Autodesk Inventor part; units mm, degrees
ref_plane "YZ Plane" through (0, 0, 0) normal (1, 0, 0) x (0, 1, 0)
ref_plane "XZ Plane" through (0, 0, 0) normal (0, 1, 0) x (-1, 0, 0)
ref_plane "XY Plane" through (0, 0, 0) normal (0, 0, 1) x (1, 0, 0)
sketch "Sketch1" plane through (0, 0, 0) normal (0, 0, 1) x (1, 0, 0)
  line L0 (57.5, 0) -> (28.75, -49.7965)
  line L1 (28.75, -49.7965) -> (-28.75, -49.7965)
  line L2 (-28.75, -49.7965) -> (-57.5, 0)
  line L3 (-57.5, 0) -> (-28.75, 49.7965)
  line L4 (-28.75, 49.7965) -> (28.75, 49.7965)
  line L5 (28.75, 49.7965) -> (57.5, 0)
  point P0 (0, 0)
  point P1 (0, 0)
  dimension "d0" = 115
extrude "Extrusion1" add sketch "Sketch1" along normal blind 159.4929
sketch "Sketch2" plane through (-28.75, -49.7965, 0) normal (0, -1, 0) x (1, 0, 0)
  line L0 (-28.75, 109.6965) -> (0, 159.4929)
  line L1 (0, 159.4929) -> (57.5, 159.4929)
  line L2 (57.5, 159.4929) -> (86.25, 109.6965)
  line L3 (86.25, 109.6965) -> (57.5, 59.9)
  line L4 (57.5, 59.9) -> (0, 59.9)
  line L5 (0, 59.9) -> (-28.75, 109.6965)
  line L6 (0, 159.4929) -> (57.5, 159.4929)
  point P0 (28.75, 0)
  point P1 (28.75, 109.6965)
  point P2 (28.75, 159.4929)
  dimension "d3" = 115
extrude "Extrusion2" add sketch "Sketch2" against normal blind 216.6673
sketch "Sketch9" plane through (0, 0, 0) normal (1, 0, 0) x (0, 1, 0)
  line L0 (0, 109.6965) -> (-49.7965, 59.9)
  line L1 (-49.7965, 109.6965) -> (0, 109.6965)
  line L2 (-49.7965, 59.9) -> (-49.7965, 109.6965)
  line L3 (-49.7965, 159.4929) -> (0, 109.6965)
  line L4 (-49.7965, 109.6965) -> (-49.7965, 159.4929)
  line L5 (-49.7965, 109.6965) -> (0, 109.6965)
  line L6 (-49.7965, 159.4929) -> (0, 109.6965)
  line L7 (0, 109.6965) -> (0, 159.4929)
  line L8 (-49.7965, 159.4929) -> (0, 159.4929)
  line L9 (0, 109.6965) -> (49.7965, 159.4929)
  line L10 (0, 159.4929) -> (49.7965, 159.4929)
  line L11 (0, 109.6965) -> (0, 159.4929)
  point P0 (0, 0)
extrude "Extrusion8" cut sketch "Sketch9" along normal through all both and the other way through all
sketch "Sketch10" plane through (0, 0, 0) normal (0, 0, -1) x (-1, 0, 0)
  circle A0 centre (0, 0) radius 25
  dimension "d24" = 50
extrude "Extrusion9" cut sketch "Sketch10" against normal blind 5
sketch "Sketch11" plane through (-28.75, 166.8708, 0) normal (0, 1, 0) x (1, 0, 0)
  line L0 (0, -59.9) -> (-28.75, -109.6965)
  line L1 (-28.75, -109.6965) -> (0, -159.4929)
  line L2 (0, -159.4929) -> (57.5, -159.4929)
  line L3 (57.5, -159.4929) -> (86.25, -109.6965)
  line L4 (86.25, -109.6965) -> (57.5, -59.9)
  line L5 (57.5, -59.9) -> (0, -59.9)
  circle A0 centre (28.75, -109.6965) radius 25
  point P0 (28.75, 0)
  point P1 (28.75, -159.4929)
  dimension "d27" = 50
extrude "Extrusion10" add sketch "Sketch11" along normal blind 5 contours A0
properties part number "link_a0" material "ABS Plastic"
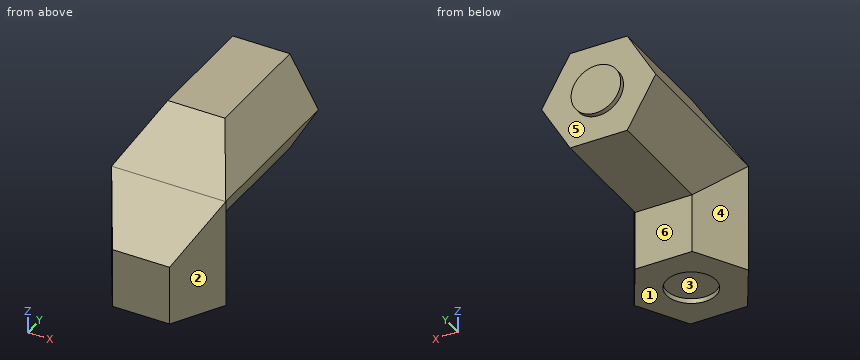
CAD build for the part. Positions are in the model's coordinates, mm. Face numbers are marked on the shaded views. A direction names the side the tool comes from. Coordinates: 2 decimals unless noted, no trailing zeros. Order: outer loops, then holes, each group sorted by start corner. A loop starts at its lowest first (then second) coordinate and runs counter-clockwise, first axis right, second up. Notation, with made-up numbers: M 18.25,25.25 L 71.25,25.25 A24 ccw 71.25,50.25 Z; hole C 40,38 d1. An arc over 180 degrees is marked long. Write each question's results on one line, items separated by ' | '. Start each with the question number.
Q1. Which spindle directions (+Z, -Z, +X, -X, +Y, -Y) get a long thin tool onto all of the face, cutting with end or side? Do the marked faces 4, 5 and 6. Say none if no direction does.
Q2. Cut at B-B (z = 42.5). List the corners of the cut face in (x, y), then the cut area to 3 significant figures.
Q3. Pull direction Y, two halves, no side cores. Call the marked faces 1, 2 and 3: +Y half, -Y half, draft (parallel to the pull), parting line (faces both ways), or undercut.
Q4. Cut at A-A (x = 0). List the corners of the cut face in (y, z), then the cut area to 3 significant figures.
Q5. Cut at C-C (y = 143). List the corners of the cut face in (x, z).
Q6. Cut at D-D (z = 63.5). List the corners of the cut face in (x, y), then the cut area to 3 significant figures.
Q7. Flat gauge pins, fed straight in: P1, Ø2, axis at x = 25, y = 63.5, coming from the -Z side; P2, Ø2, axis at y = 99, z = 92.5, coming from the +X side; P3, Ø3, axis at x = 37, z = 99, coming from the +Y side; P4, Ø10, axis at x = -30.5, y = 9, coming from the -Z side. Where does each tip first touch, or does it go through?
Q8. Drill centre lines: probe 1 along Y at (x, z) = (0, 2.4); probe 2 along Z at (x, y) = (8, 55.5); probe 3 along Y at (x, z) = (23, 26). Where is each one in solid material? Low to high. Write a range as from..to.
Found:
1) face 4: -Z, -X, +Y | face 5: +Y | face 6: -Z, +X, -X, +Y
2) outline: M -57.5,0 L -28.75,-49.8 L 28.75,-49.8 L 57.5,0 L 28.75,49.8 L -28.75,49.8 Z | area: 8,590 mm²
3) face 1: draft | face 2: -Y half | face 3: undercut
4) outline: M -49.8,0 L -25,0 L -25,5 L 25,5 L 25,0 L 49.8,0 L 49.8,59.9 L 166.87,59.9 L 166.87,84.7 L 171.87,84.7 L 171.87,134.7 L 166.87,134.7 L 166.87,159.49 L 49.8,159.49 L 0,109.7 L -49.8,59.9 Z | area: 22,600 mm²
5) outline: M -57.5,109.7 L -28.75,59.9 L 28.75,59.9 L 57.5,109.7 L 28.75,159.49 L -28.75,159.49 Z
6) outline: M -57.5,0 L -30.83,-46.2 L 30.83,-46.2 L 57.5,0 L 30.83,46.2 L 30.83,166.87 L -30.83,166.87 L -30.83,46.2 Z | area: 15,600 mm²
7) P1: z = 59.9 | P2: x = 48.15 | P3: y = 166.87 | P4: z = 0
8) probe 1: -49.8..-25, 25..49.8 | probe 2: 59.9..159.49 | probe 3: -49.8..49.8
